Work out the finished part from the listing and answer in its coordinate system (mm). Face numbers are marked on the shaded views. A direction names the side the tool comes from. Give positions to 0.01 mm unless a question says otherwise; leave off trailing zeros. Write each loop counter-clockwise with the first axis right and the second up, starting at its lowest first coordinate (ties: lowest second). Pieces come first, ordered by that corner, then holes. Notation, with made-up numbers: (-20.5, -40) -> (15.5, -40) arc R20 ccw to (15.5, -10) -> close; hole circle Ø4 at (14, -26). An arc over 180 degrees is marked (long way). Write item = value, one per line. Start each with the question number.
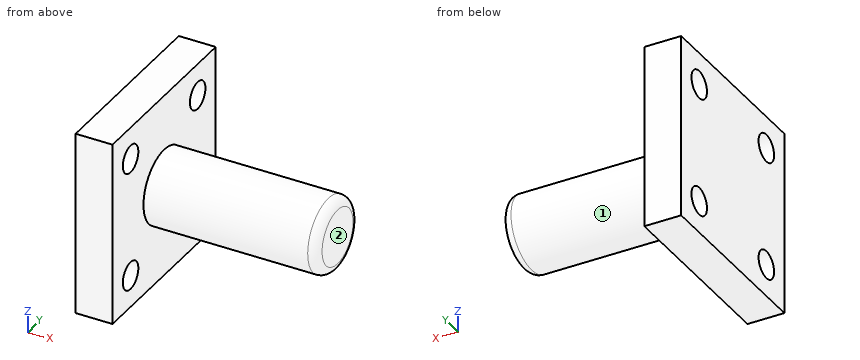
from build123d import *

# Parameters (mm, degrees)
SKETCH1_W             = 20
SKETCH1_H             = 20
BOSS_EXTRUDE1_DEPTH   = 4
SKETCH2_R             = 4
BOSS_EXTRUDE2_DEPTH   = 18.8
F_3_0MM_DOWEL_HOLE1_D = 3
FILLET1_R             = 1


with BuildPart() as part:
    # Sketch1 → Boss-Extrude1 (new body)
    with BuildSketch(Plane(origin=(0, 0, 0), x_dir=(0, 0, -1), z_dir=(1, 0, 0))):
        Rectangle(SKETCH1_W, SKETCH1_H)
    extrude(amount=BOSS_EXTRUDE1_DEPTH)

    # Sketch2 → Boss-Extrude2 (add)
    with BuildSketch(Plane(origin=(4, 0, 0), x_dir=(0, 0, -1), z_dir=(1, 0, 0))):
        with Locations(Location((0, 0, 0), (0, 0, 180))):
            Circle(SKETCH2_R)
    extrude(amount=BOSS_EXTRUDE2_DEPTH)

    # Ø3.0mm Dowel Hole1 (through all)
    with Locations(Plane.ZY):
        with Locations((-6.5, -6.5), (-6.5, 6.5), (6.5, 6.5), (6.5, -6.5)):
            Hole(F_3_0MM_DOWEL_HOLE1_D / 2)

    # Fillet1
    fillet1_edges = [part.edges().sort_by_distance(p)[0] for p in [
        (22.8, 0, -4),
    ]]
    fillet(fillet1_edges, radius=FILLET1_R)


solid = part.part
(1) For the marked faces 1 and 2, determine the directions among +Z, -Z, +X, -X, +Y, -Y from which every point of the face is accessible in a straight line to the end or side of a thin tool.
(2) A cutting plane is placed at D-D, the plane x = 17.5. Write down the section's boundary in (y, z).
(3) Find the intervals of material crossed by line 1 along Y through (x, z) = (2.2, -6.5); line 2 along X through (y, z) = (7.75, -1.75); line 3 along Y through (x, z) = (15.5, -0.25), in increasing order.
(4) A cutting plane is placed at C-C, the plane y = 0. Write down the section's boundary in (x, z).
(5) Each of these flat-tipped pins is pushed along its axis until it touches: pin 1 (3 mm diameter, centred on x = 15, y = -2.5, fed in from -Z); pin 2 (3 mm diameter, centred on x = 6, z = 4.5, fed in from -Y); pin 3 (6 mm diameter, centred on x = 14, y = -1, fed in from -Z). Where does it stop, or does it pass through?
(6) A cutting plane is placed at A-A, the plane z = 6.5. Write down the section's boundary in (x, y).
Results list:
q1.face_1 = +X
q1.face_2 = +Z, -Z, +X, +Y, -Y
q2.outline = circle Ø8 at (0, 0)
q3.line_1 = -10 to -8, -5 to 5, 8 to 10
q3.line_2 = 0 to 4
q3.line_3 = -3.99 to 3.99
q4.outline = (0, -10) -> (4, -10) -> (4, -4) -> (21.8, -4) arc R1 ccw to (22.8, -3) -> (22.8, 3) arc R1 ccw to (21.8, 4) -> (4, 4) -> (4, 10) -> (0, 10) -> close
q5.pin_1 = -3.87
q5.pin_2 = -2.65
q5.pin_3 = -4
q6.outline = (0, -10) -> (4, -10) -> (4, -8) -> (0, -8) -> close; (0, -5) -> (4, -5) -> (4, 5) -> (0, 5) -> close; (0, 8) -> (4, 8) -> (4, 10) -> (0, 10) -> close
